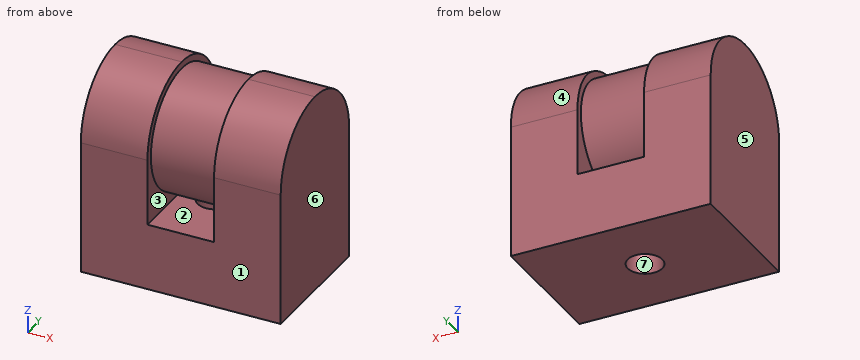
```python
from build123d import *

# Parameters (mm, degrees)
SZKIC1_W                    = 30
SZKIC1_H                    = 20
SZKIC1_R                    = 2.6
DODANIE_WYCI_GNI_CIE1_DEPTH = 10
SZKIC2_W                    = 10
SZKIC2_H                    = 20
DODANIE_WYCI_GNI_CIE2_DEPTH = 20
SZKIC3_R                    = 9
DODANIE_WYCI_GNI_CIE3_DEPTH = 10
ZAOKR_GLENIE1_R             = 10


with BuildPart() as part:
    # Szkic1 → Dodanie-wyciągnięcie1 (new body)
    with BuildSketch(Plane.XY):
        with Locations((15, 10)):
            Rectangle(SZKIC1_W, SZKIC1_H)
        with Locations((15, 10)):
            Circle(SZKIC1_R, mode=Mode.SUBTRACT)
    extrude(amount=DODANIE_WYCI_GNI_CIE1_DEPTH)

    # Szkic2 → Dodanie-wyciągnięcie2 (add)
    with BuildSketch(Plane.XY.offset(10)):
        with Locations((5, 10)):
            Rectangle(SZKIC2_W, SZKIC2_H)
        with Locations((25, 10)):
            Rectangle(SZKIC2_W, SZKIC2_H)
    extrude(amount=DODANIE_WYCI_GNI_CIE2_DEPTH)

    # Szkic3 → Dodanie-wyciągnięcie3 (add)
    with BuildSketch(Plane(origin=(10, 0, 0), x_dir=(0, 0, -1), z_dir=(1, 0, 0))):
        with Locations(Location((-20, 10, 0), (0, 0, 270))):
            Circle(SZKIC3_R)
    extrude(amount=DODANIE_WYCI_GNI_CIE3_DEPTH)

    # Zaokrąglenie1
    zaokr_glenie1_edges = [part.edges().sort_by_distance(p)[0] for p in [
        (25, 0, 30),
        (5, 0, 30),
        (25, 20, 30),
        (5, 20, 30),
    ]]
    fillet(zaokr_glenie1_edges, radius=ZAOKR_GLENIE1_R - 0.0001)  # a hair under: the kernel refuses the full size


solid = part.part
```
Build history of the part. All positions in model axes, mm. Face numbers are marked on the shaded views. A direction names the side the tool comes from. Round coordinates to 2 decimals unless told otherwise and drop trailing zeros. Write each loop counter-clockwise with the first axis right and the second up, starting at its lowest first coordinate (ties: lowest second). Pieces come first, ordered by that corner, then holes.
1) Mould opens along X. For the marked faces 4, 5, 6 and 7 say: +X half, -X half, draft (parallel to the pull), parting line (faces both ways), or undercut.
2) 3-axis set-ups, long thin cutter, end or side, ignore diameter. For the marked faces 1, 2 and 3: which of +Z, -Z, +X, -X, +Y, -Y reach the whole face in a straight line?
3) Band-saw the part on C-C, the plane y = 15. List the corners of the cut face in (x, z), and give its area (3 significant figures).
4) Band-saw the part on B-B, the plane z = 3. List the corners of the cut face in (x, y), and give its area (3 significant figures).
5) Drill centre lines: probe 1 along Y at (x, z) = (15, 5.5); probe 2 along X at (y, z) = (1.25, 15); probe 3 along Z at (x, y) = (3.75, 18). Where is each one in solid material? Low to high.
6) Pin check, flat tips, straight feed: pin 1 (8.5 mm diameter, centred on x = 15, y = 10, fed in from +Z); pin 2 (3 mm diameter, centred on x = 14, z = 17, fed in from +Y); pin 3 (4 mm diameter, centred on x = 15.5, z = 18, fed in from +Y). Stop position of each tip, or through.
7) Band-saw the part on A-A, the plane x = 15. List the corners of the cut face in (y, z).
Ans:
1. face 4: draft
1. face 5: -X half
1. face 6: +X half
1. face 7: undercut
2. face 1: +Z, -Z, +X, -X, -Y
2. face 2: +Y, -Y
2. face 3: none
3. outline: (0, 0) - (30, 0) - (30, 28.66) - (20, 28.66) - (20, 27.48) - (10, 27.48) - (10, 28.66) - (0, 28.66) - close; hole (10, 10) - (20, 10) - (20, 12.52) - (10, 12.52) - close
3. area: 823 mm2
4. outline: (0, 0) - (30, 0) - (30, 20) - (0, 20) - close; hole circle Ø5.2 at (15, 10)
4. area: 579 mm2
5. probe 1: y = 0 to 7.4, 12.6 to 20
5. probe 2: x = 0 to 10, 20 to 30
5. probe 3: z = 0 to 26
6. pin 1: stops at z = 29
6. pin 2: stops at y = 18.87
6. pin 3: stops at y = 19
7. outline: (0, 0) - (7.4, 0) - (7.4, 10) - (0, 10) - close; circle Ø18 at (10, 20); (12.6, 0) - (20, 0) - (20, 10) - (12.6, 10) - close
